The figure shows three views and two pictorial views of one solid part (mm, origin at its lowest corner). Answer the questions. Round coordinates to 2 decimals unless told otherwise and drop trailing zeros. Order: outer loops, then holes, each group sorted by start corner. A loop starts at its lowest first (then second) coordinate and runs counter-clockwise, first axis right, second up. Notation, with made-up numbers: (-14, 43.25) - (-6, 43.25) arc R5 ccw to (-6, 50.25) - close; hole circle Ø8 at (39, 24.5). An arc over 180 degrees is marked (long way). One line per question, with ' | ' between items. Start each with the question number.
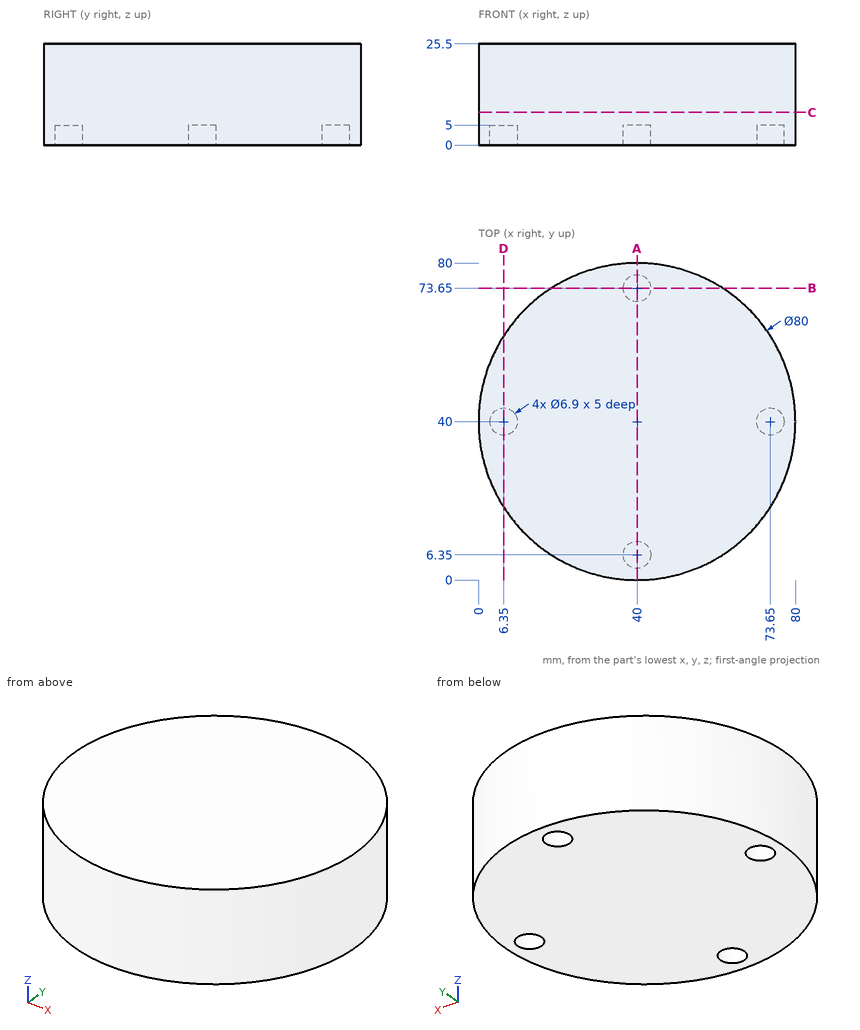
1) Section C-C on z = 8.25 is taken. Give the vertices of the cut face in (x, y).
2) Straight lines are drawn through the part: line 1 (Y direction, x = 40, z = 2.8); line 2 (Y direction, x = 55, z = 15); line 3 (X direction, y = 73.65, z = 1.6). For each, find the intervals that lie inside material, in ascending order.
3) Section B-B on y = 73.65 is taken. Give the vertices of the cut face in (x, z), and give its area (3 significant figures).
4) Section A-A on x = 40 is taken. Give the vertices of the cut face in (y, z).
5) Flat-ended cylindrical pins translate along their axes: pin 1 (3.5 mm diameter, centred on x = 38.5, y = 6.5, fed in from -Z); pin 2 (12 mm diameter, centred on y = 15.5, z = 5.5, fed in from -X); pin 3 (4 mm diameter, centred on y = 28.5, z = 7.5, fed in from -X). Find the tip coordinate at first contact, or state that the pin passes through.
Recorded:
1) outline: circle Ø80 at (40, 40)
2) line 1: y = 0 to 2.9, 9.8 to 70.2, 77.1 to 80 | line 2: y = 2.92 to 77.08 | line 3: x = 18.37 to 36.55, 43.45 to 61.63
3) outline: (18.37, 0) - (36.55, 0) - (36.55, 5) - (43.45, 5) - (43.45, 0) - (61.63, 0) - (61.63, 25.5) - (18.37, 25.5) - close | area: 1,070 mm²
4) outline: (0, 0) - (2.9, 0) - (2.9, 5) - (9.8, 5) - (9.8, 0) - (70.2, 0) - (70.2, 5) - (77.1, 5) - (77.1, 0) - (80, 0) - (80, 25.5) - (0, 25.5) - close
5) pin 1: stops at z = 5 | pin 2: stops at x = 4.54 | pin 3: stops at x = 1.14
